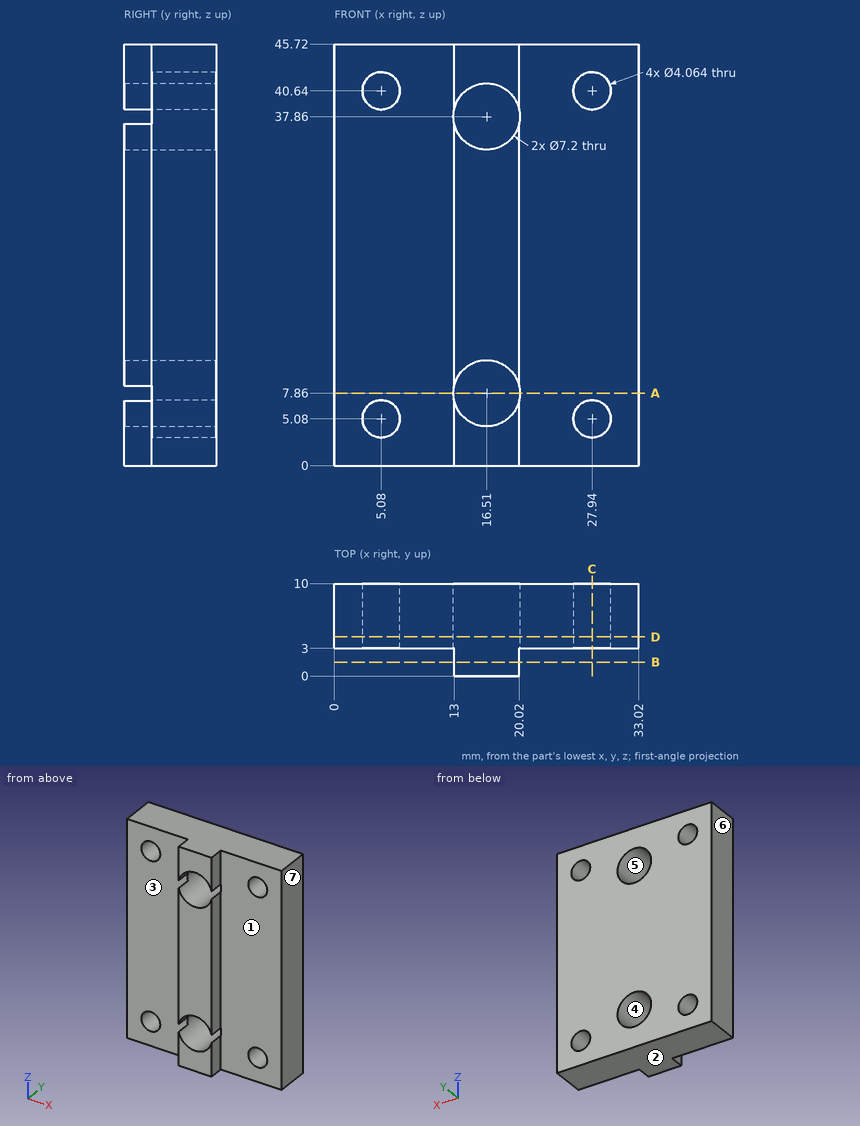
Print and shaded views of the part. All mm, measured from the part's lowest x, y and z. A direction names the side the tool comes from. Give positions to 0.01 mm unless a question says otherwise; leave off trailing zeros. Loops run counter-clockwise (first coordinate to the right, second up) from the corner with the lowest first, then second, coordinate; pieces in that order, holes last. Notation, with made-up numbers: (50, 36) -> (93, 36) arc R36 cw to (93, 73) -> close; hole circle Ø1 at (-40, 43.25). An arc over 180 degrees is marked (long way). Use a Markdown table: item, result.
1. Slice it at D-D (y = 4.25). List the corners of the cut face in (x, z).
Check result:
| item | result |
|---|---|
| outline | (0, 0) -> (33.02, 0) -> (33.02, 45.72) -> (0, 45.72) -> close; hole circle Ø4.06 at (5.08, 5.08); hole circle Ø4.06 at (5.08, 40.64); hole circle Ø7.2 at (16.51, 7.86); hole circle Ø7.2 at (16.51, 37.86); hole circle Ø4.06 at (27.94, 5.08); hole circle Ø4.06 at (27.94, 40.64) |
2. Flat gauge pins, fed straight in: pin 1 (8.5 mm diameter, centred on x = 16.51, z = 37.86, fed in from +Y); pin 2 (6.5 mm diameter, centred on x = 5.5, z = 20, fed in from -Y); pin 3 (2.5 mm diameter, centred on y = 1, z = 27, fed in from +X); pin 4 (0.9 mm diameter, centred on y = 1.5, z = 16.5, fed in from -X). Where does each tip first touch, or does it go through?
Check result:
| item | result |
|---|---|
| pin 1 | stops at y = 10 |
| pin 2 | stops at y = 3 |
| pin 3 | stops at x = 20.02 |
| pin 4 | stops at x = 13 |
3. Slice it at C-C (x = 27.94). List the corners of the cut face in (y, z), plus the area to 3 significant figures.
Check result:
| item | result |
|---|---|
| outline | (3, 0) -> (10, 0) -> (10, 3.05) -> (3, 3.05) -> close; (3, 7.11) -> (10, 7.11) -> (10, 38.61) -> (3, 38.61) -> close; (3, 42.67) -> (10, 42.67) -> (10, 45.72) -> (3, 45.72) -> close |
| area | 263 mm^2 |
4. Wall check: L1, parallel to Z at x = 27.94, y = 5; L2, parallel to Z at x = 16.51, y = 6; L3, parallel to X at y = 5.5, z = 40.64. Give the ranges that are in metal, low to high. Write a range as [from, to].
Check result:
| item | result |
|---|---|
| L1 | z = [0, 3.05], [7.11, 38.61], [42.67, 45.72] |
| L2 | z = [0, 4.26], [11.46, 34.26], [41.46, 45.72] |
| L3 | x = [0, 3.05], [7.11, 14.22], [18.8, 25.91], [29.97, 33.02] |
5. Slice it at B-B (y = 1.5). List the corners of the cut face in (x, z), plus the area to 3 significant figures.
Check result:
| item | result |
|---|---|
| outline | (13, 0) -> (20.02, 0) -> (20.02, 7.06) arc R3.6 cw to (13, 7.06) -> close; (13, 8.66) arc R3.6 cw to (20.02, 8.66) -> (20.02, 37.06) arc R3.6 cw to (13, 37.06) -> close; (13, 38.66) arc R3.6 cw to (20.02, 38.66) -> (20.02, 45.72) -> (13, 45.72) -> close |
| area | 240 mm^2 |
6. Mould opens along X. For the marked faces 4, 5, 6 and 7 say: pulls with the +X half, pulls with the -X half, needs draft (parallel to the pull), parting line crosses it, or undercut.
Check result:
| item | result |
|---|---|
| face 4 | undercut |
| face 5 | undercut |
| face 6 | pulls with the -X half |
| face 7 | pulls with the +X half |
7. Which spindle directions (+Z, -Z, +X, -X, +Y, -Y) get a long thin tool onto all of the face, cutting with end or side? Do the marked faces 1, 2 and 3. Say none if no direction does.
Check result:
| item | result |
|---|---|
| face 1 | +Z, -Z, +X, -Y |
| face 2 | -Z, +X, -X, +Y, -Y |
| face 3 | +Z, -Z, -X, -Y |
8. Slice it at A-A (z = 7.86). List the corners of the cut face in (x, y), plus the area to 3 significant figures.
Check result:
| item | result |
|---|---|
| outline | (0, 3) -> (12.91, 3) -> (12.91, 10) -> (0, 10) -> close; (20.11, 3) -> (33.02, 3) -> (33.02, 10) -> (20.11, 10) -> close |
| area | 181 mm^2 |
